from build123d import *


with BuildPart() as part:
    # Sweep1: sweep along a path in Sketch2
    with BuildLine(Plane(origin=(0, 0, 0), x_dir=(0, 0, -1), z_dir=(1, 0, 0))) as sweep1_path:
        Line((0, 0), (0, 77.75))
        ThreePointArc((0, 77.75), (0.878679656, 79.871320344), (3, 80.75))
        Line((3, 80.75), (14.75, 80.75))
    # Sketch1 → Sweep1 (sweep)
    with BuildSketch(Plane(origin=(0, 0, 0), x_dir=(1, 0, 0), z_dir=(0, 1, 0))):
        Polygon((0.866025404, 0), (0.433012702, 0.75), (-0.433012702, 0.75), (-0.866025404, 0), (-0.433012702, -0.75), (0.433012702, -0.75), align=None)
    sweep(path=sweep1_path.line)


solid = part.part
Check sheet for the modelled part. Datum: model origin and axes. Units: mm. Coordinates: 2 decimals unless noted, no trailing zeros. Loops run counter-clockwise (first coordinate to the right, second up) from the corner with the lowest first, then second, coordinate; pieces in that order, holes last. Notation, with made-up numbers: (42, -18.5) -> (52, -18.5) arc R23 ccw to (52, 1.5) -> close; hole circle Ø6 at (59.25, 66). An arc over 180 degrees is marked (long way). Write item = value, one per line. Start each with the question number.
1. Section check C-C on z = -7.5. Record the cut outline in (x, y), then the cut area to 3 significant figures.
2. Section check A-A on x = -0.15. Record the cut outline in (y, z), then the cut area to 3 significant figures.
3. Depth check by flat-ended pin: P1, Ø0.7, axis at x = 0, y = 37.5, coming from the -Z side; P2, Ø1, axis at x = 0, z = -9, coming from the -Y side; P3, Ø4, axis at y = 58.5, z = -3.5, coming from the -X side. Enter the tip coordinate at first touch or a pass-through.
4. Draft check along Z on faces 1 (the flat face through (0, 0, 0)), 2 (the cylindrical face through (0, 80, 0)), 3 (the cylindrical face through (-0.01, 79.32, -1.39)). Enter one of: released by +Z, released by -Z, zero draft, split by the parting line, or undercut.
5. Material ranges on line 1 (Z direction, x = -0.35, y = 29.5); line 2 (Y direction, x = -0.1, z = -7.25); line 3 (Z direction, x = -0.65, y = 33), recorded low to high.
6. Section check B-B on y = 39.5. Record the cut outline in (x, z).
Responses:
q1.outline = (-0.87, 80.75) -> (-0.43, 80) -> (0.43, 80) -> (0.87, 80.75) -> (0.43, 81.5) -> (-0.43, 81.5) -> close
q1.area = 1.95 mm2
q2.outline = (0, -0.75) -> (77.75, -0.75) arc R2.25 cw to (80, -3) -> (80, -14.75) -> (81.5, -14.75) -> (81.5, -3) arc R3.75 ccw to (77.75, 0.75) -> (0, 0.75) -> close
q2.area = 141 mm2
q3.P1 = -0.75
q3.P2 = 80
q3.P3 = through
q4.face_1 = zero draft
q4.face_2 = released by +Z
q4.face_3 = released by -Z
q5.line_1 = -0.75 to 0.75
q5.line_2 = 80 to 81.5
q5.line_3 = -0.37 to 0.37
q6.outline = (-0.87, 0) -> (-0.43, -0.75) -> (0.43, -0.75) -> (0.87, 0) -> (0.43, 0.75) -> (-0.43, 0.75) -> close
